Here's how the part is built. I have some questions about the finished solid (model axes, mm). Coordinates: 2 decimals unless noted, no trailing zeros. Write each loop counter-clockwise with the first axis right and the second up, starting at its lowest first coordinate (ties: lowest second). Pieces come first, ordered by that corner, then holes.
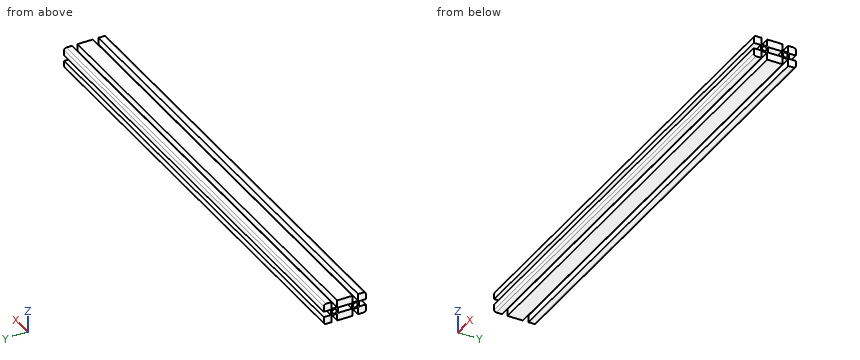
```python
from build123d import *

# Parameters (mm, degrees)
F1_DEPTH = 335
F2_W     = 20
F2_H     = 8
F2_R     = 3.4
F3_DEPTH = 670
F4_R     = 3


with BuildPart() as f1:
    # F0 (on Right) → F1 (new body, symmetric)
    with BuildSketch(Plane.YZ):
        Polygon((30, 4), (30, 15), (19, 15), (19, 5), (11, 5), (11, 15), (-11, 15), (-11, 5), (-19, 5), (-19, 15), (-30, 15), (-30, 4), (-20, 4), (-20, -4), (-30, -4), (-30, -15), (-19, -15), (-19, -5), (-11, -5), (-11, -15), (11, -15), (11, -5), (19, -5), (19, -15), (30, -15), (30, -4), (20, -4), (20, 4), align=None)
    extrude(amount=F1_DEPTH, both=True)

    # F2 (on face) → F3 (cut)
    with BuildSketch(Plane.YZ.offset(335)):
        Rectangle(F2_W, F2_H)
        with Locations((-15, 0)):
            Circle(F2_R)
        with Locations((15, 0)):
            Circle(F2_R)
    extrude(amount=-F3_DEPTH, mode=Mode.SUBTRACT)

    # F4
    f4_edges = [f1.edges().sort_by_distance(p)[0] for p in [
        (0, -30, 15),
        (0, -30, -15),
        (0, 30, 15),
        (0, 30, -15),
    ]]
    fillet(f4_edges, radius=F4_R)


solid = f1.part
```
1) I need wall thicknesses on probe 1 along Y at (x, z) = (-20.5, -12.5); probe 2 along Y at (x, z) = (99.5, -2.75); probe 3 along Y at (x, z) = (45, 2.5). Which ranges of each line are inside material? Lowest first, please.
Values follow:
probe 1: y = -29.96 to -19, -11 to 11, 19 to 29.96
probe 2: y = -20 to -17, -13 to -10, 10 to 13, 17 to 20
probe 3: y = -20 to -17.3, -12.7 to -10, 10 to 12.7, 17.3 to 20
2) Imagine slicing it at A-A on y = 1. Please give me the cut outline in (x, z), then the cut area to 3 significant figures.
Values follow:
outline: (-335, -15) - (335, -15) - (335, -4) - (-335, -4) - close; (-335, 4) - (335, 4) - (335, 15) - (-335, 15) - close
area: 14,700 mm2
3) Will these pins go through, and if not, where does the flat tip stop? pin 1 (4 mm diameter, centred on x = -51, y = 15, fed in from +Z); pin 2 (4 mm diameter, centred on x = 113.5, z = 1, fed in from -Y); pin 3 (2.5 mm diameter, centred on x = 29, z = -0.5, fed in from +Y).
Values follow:
pin 1: stops at z = 5
pin 2: stops at y = -20
pin 3: stops at y = 20
4) Imagine slicing it at B-B on x = -200.5. Count the separate pieces of the cut face and the enclosed holes in it, then the cut area to 3 significant figures.
Values follow:
separate pieces: 1
enclosed holes: 3
area: 1,080 mm2
